Verification items for this drawing (mm, ordinates from the low corner). A direction names the side the tool comes from. Round coordinates to 2 decimals unless told otherwise and drop trailing zeros. Order: outer loops, then holes, each group sorted by start corner. A loop starts at its lowest first (then second) coordinate and runs counter-clockwise, first axis right, second up. Notation, with made-up numbers: (67.25, 51.25) - (86.25, 51.25) arc R16 ccw to (86.25, 64.25) - close; hole circle Ø4 at (57.25, -4.5). An arc over 180 degrees is marked (long way). Use a Markdown table: item, result. Add a question column.
(1) Section check B-B on z = 3.75. Record the boundary of the cut face in (x, y).
(2) Thickness scan on line 1 along X through (y, z) = (2, 3.3); line 2 along Y through (x, z) = (15, 5.75). Record the ranges inside material, lowest first. Write a range as [from, to].
(3) Mould release check, pull along X, two halves, no side actions. Record for the marked faces 4, 5 and 6: released by +X, released by -X, zero draft, split by the parting line, or undercut.
(4) Gauge pin test, flat end, axial feed: P1, Ø1.8, axis at x = 33, z = 2.5, coming from the -Y side. Record the tip position at first contact, or that the pin passes through.
(5) Section check A-A on y = 8.5. Record the boundary of the cut face in (x, z), then the cut area to 3 significant figures.
(6) Access from +Z, -Z, +X, -X, +Y, -Y to the whole of each face (thin tool, end or side, straight path). Record for the marked faces 1, 2 and 3.
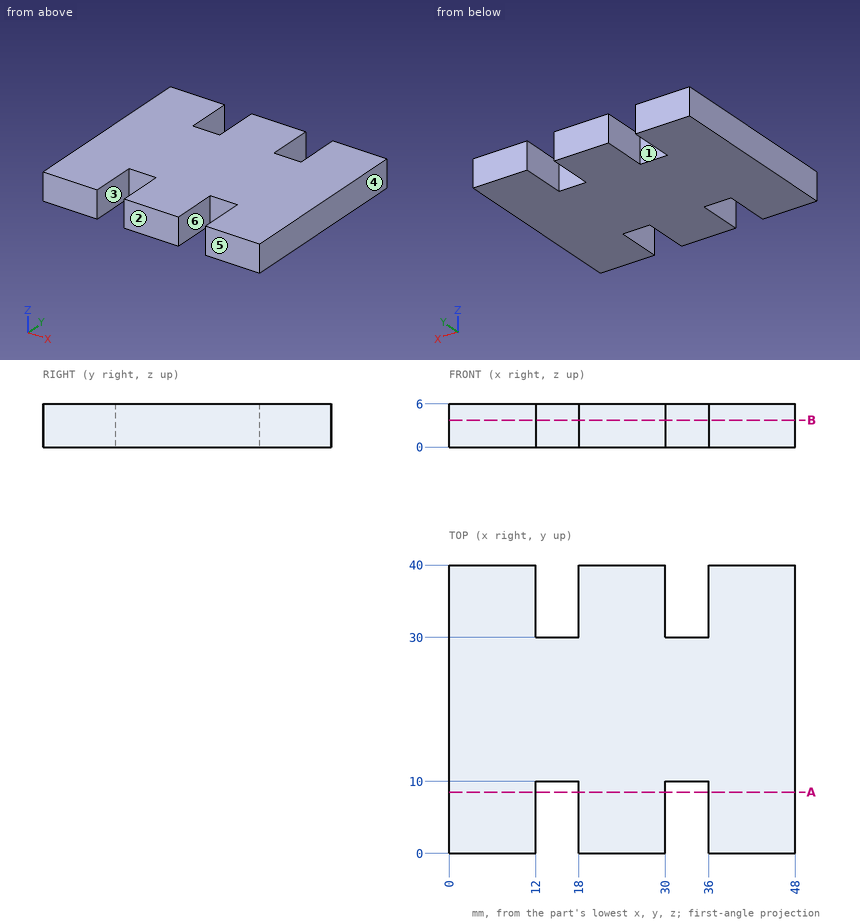
Check sheet entries:
| question | item | result |
|---|---|---|
| 1 | outline | (0, 0) - (12, 0) - (12, 10) - (18, 10) - (18, 0) - (30, 0) - (30, 10) - (36, 10) - (36, 0) - (48, 0) - (48, 40) - (36, 40) - (36, 30) - (30, 30) - (30, 40) - (18, 40) - (18, 30) - (12, 30) - (12, 40) - (0, 40) - close |
| 2 | line 1 | x = [0, 12], [18, 30], [36, 48] |
| 2 | line 2 | y = [10, 30] |
| 3 | face 4 | released by +X |
| 3 | face 5 | zero draft |
| 3 | face 6 | undercut |
| 4 | P1 | stops at y = 10 |
| 5 | outline | (0, 0) - (12, 0) - (12, 6) - (0, 6) - close; (18, 0) - (30, 0) - (30, 6) - (18, 6) - close; (36, 0) - (48, 0) - (48, 6) - (36, 6) - close |
| 5 | area | 216 mm2 |
| 6 | face 1 | +Z, -Z, +Y |
| 6 | face 2 | +Z, -Z, +X, -X, -Y |
| 6 | face 3 | +Z, -Z, -Y |
